```python
from build123d import *

# Parameters (mm, degrees)
SKETCH_1_R                   = 5
EXTRUDE_1_DEPTH              = 10.5
EXTRUDE_1_DEPTH_BACK         = 10.5
EXTRUDE_3_DEPTH              = 4.5
EXTRUDE_3_DEPTH_BACK         = 4.5
SKETCH_7_R                   = 6
EXTRUDE_4_DEPTH              = 3
SKETCH_8_R                   = 6
EXTRUDE_5_DEPTH              = 3
SKETCH_9_R                   = 9.5
CUT_EXTRUDE_1_DEPTH          = 7
SKETCH_10_R                  = 8.5
CUT_EXTRUDE_2_DEPTH          = 9
HOLE_WIZARD_M4_1_D           = 3.3
SKETCH_22_W                  = 47.656916312
SKETCH_22_H                  = 14.908676054
CUT_EXTRUDE_3_DEPTH          = 1111
SKETCH_23_R                  = 9.5
SKETCH_23_R_2                = 8.5
EXTRUDE_6_DEPTH              = 2
HOLE_WIZARD_M3_1_D           = 3.2
HOLE_WIZARD_M3_1_CBORE_D     = 6.5
HOLE_WIZARD_M3_1_CBORE_DEPTH = 3.4
PATTERN_CIRCULAR_1_COUNT     = 6
HOLE_WIZARD_M3_2_D           = 3.2
HOLE_WIZARD_M3_2_CBORE_D     = 6.5
HOLE_WIZARD_M3_2_CBORE_DEPTH = 3.4
PATTERN_LINEAR_1_COUNT       = 3
PATTERN_LINEAR_1_PITCH       = 70
PATTERN_LINEAR_1_COUNT_DIR2  = 2
PATTERN_LINEAR_1_PITCH_DIR2  = 10
SKETCH_31_R                  = 3.25
EXTRUDE_7_DEPTH              = 5.5


with BuildPart() as part:
    # Sketch 1 → Extrude 1 (new body, two sides)
    with BuildSketch(Plane(origin=(0, 0, 0), x_dir=(1, 0, 0), z_dir=(0, 1, 0))) as extrude_1_sk:
        Circle(SKETCH_1_R)
    extrude(amount=EXTRUDE_1_DEPTH)
    extrude(extrude_1_sk.sketch, amount=-EXTRUDE_1_DEPTH_BACK)

    # Sketch 6 → Extrude 3 (add, two sides)
    with BuildSketch(Plane(origin=(0, 0, 0), x_dir=(1, 0, 0), z_dir=(0, 1, 0))) as extrude_3_sk:
        with BuildLine():
            Line((-12.5, 0), (-12.5, -260))
            ThreePointArc((-12.5, -260), (0, -272.5), (12.5, -260))
            Line((12.5, -260), (12.5, 0))
            ThreePointArc((12.5, 0), (0, 12.5), (-12.5, 0))
        make_face()
    extrude(amount=EXTRUDE_3_DEPTH)
    extrude(extrude_3_sk.sketch, amount=-EXTRUDE_3_DEPTH_BACK)

    # Sketch 7 → Extrude 4 (add)
    with BuildSketch(Plane.XZ.offset(4.5)):
        Circle(SKETCH_7_R)
    extrude(amount=EXTRUDE_4_DEPTH)

    # Sketch 8 → Extrude 5 (add)
    with BuildSketch(Plane(origin=(0, 4.5, 0), x_dir=(1, 0, 0), z_dir=(0, 1, 0))):
        Circle(SKETCH_8_R)
    extrude(amount=EXTRUDE_5_DEPTH)

    # Sketch 9 → Cut-Extrude 1 (cut)
    with BuildSketch(Plane.XZ.offset(4.5)):
        with Locations((0, 250)):
            Circle(SKETCH_9_R)
    extrude(amount=-CUT_EXTRUDE_1_DEPTH, mode=Mode.SUBTRACT)

    # Sketch 10 → Cut-Extrude 2 (cut, through all)
    with BuildSketch(Plane.XZ.offset(-2.5)):
        with Locations((0, 250)):
            Circle(SKETCH_10_R)
    extrude(amount=-CUT_EXTRUDE_2_DEPTH, mode=Mode.SUBTRACT)

    # Hole Wizard M4 _ _ _ _1 (through all)
    with Locations(Plane(origin=(0, -10.5, 0), x_dir=(-1, 0, 0), z_dir=(0, -1, 0))):
        with Locations((0, 0)):
            Hole(HOLE_WIZARD_M4_1_D / 2)

    # Sketch 22 → Cut-Extrude 3 (cut, symmetric)
    with BuildSketch(Plane.XY):
        with Locations((0.455125877, 8.454338027)):
            Rectangle(SKETCH_22_W, SKETCH_22_H)
    extrude(amount=CUT_EXTRUDE_3_DEPTH, both=True, mode=Mode.SUBTRACT)

    # Sketch 23 → Extrude 6 (add)
    with BuildSketch(Plane.XZ.offset(4.5)):
        with Locations((0, 250)):
            Circle(SKETCH_23_R)
        with Locations((0, 250)):
            Circle(SKETCH_23_R_2, mode=Mode.SUBTRACT)
    extrude(amount=-EXTRUDE_6_DEPTH)

    # Hole Wizard M3 _ _ _ _ _ _1 (through all)
    with Locations(Plane(origin=(0, -4.5, 0), x_dir=(-1, 0, 0), z_dir=(0, -1, 0))):
        with Locations((6.75, -261.691342951)):
            hole_wizard_m3_1 = CounterBoreHole(HOLE_WIZARD_M3_1_D / 2, HOLE_WIZARD_M3_1_CBORE_D / 2, HOLE_WIZARD_M3_1_CBORE_DEPTH)

    # Pattern Circular 1: Hole Wizard M3 _ _ _ _ _ _1 ×6 about axis, 2 skipped
    pattern_circular_1_axis = Axis((0, -2.5, 250), (0, -1, 0))
    add([hole_wizard_m3_1.rotate(pattern_circular_1_axis, i * 360 / PATTERN_CIRCULAR_1_COUNT) for i in range(1, PATTERN_CIRCULAR_1_COUNT) if i not in (1, 4)], mode=Mode.SUBTRACT)

    # Hole Wizard M3 _ _ _ _ _ _2 (through all)
    with Locations(Plane(origin=(0, -4.5, 0), x_dir=(-1, 0, 0), z_dir=(0, -1, 0))):
        with Locations((5, -15)):
            hole_wizard_m3_2 = CounterBoreHole(HOLE_WIZARD_M3_2_D / 2, HOLE_WIZARD_M3_2_CBORE_D / 2, HOLE_WIZARD_M3_2_CBORE_DEPTH)

    # Pattern Linear 1: Hole Wizard M3 _ _ _ _ _ _2 3 × 2
    with Locations(*[(j * PATTERN_LINEAR_1_PITCH_DIR2, 0, i * PATTERN_LINEAR_1_PITCH) for i in range(PATTERN_LINEAR_1_COUNT) for j in range(PATTERN_LINEAR_1_COUNT_DIR2) if (i, j) != (0, 0)]):
        add(hole_wizard_m3_2, mode=Mode.SUBTRACT)

    # Sketch 31 → Extrude 7 (add)
    with BuildSketch(Plane.XZ.offset(4.5)):
        with Locations((5, 15)):
            Circle(SKETCH_31_R)
        with Locations((-5, 15)):
            Circle(SKETCH_31_R)
    extrude(amount=-EXTRUDE_7_DEPTH)


solid = part.part
```
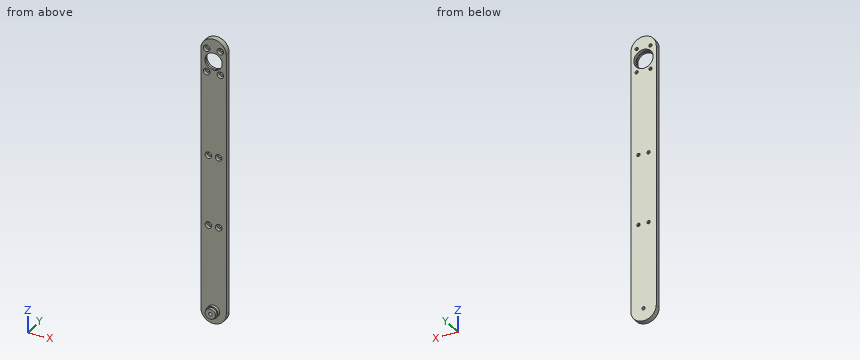
Work out the finished part from the listing and answer in its coordinate system (mm). Give positions to 0.01 mm unless a question says otherwise; leave off trailing zeros. Order: outer loops, then holes, each group sorted by start corner. A loop starts at its lowest first (then second) coordinate and runs counter-clockwise, first axis right, second up.
1. Each of these flat-tipped pins is pushed along its axis until it touches: P1, Ø3.5, axis at x = 5, z = 155, coming from the -Y side; P2, Ø4, axis at x = 0.5, z = 185, coming from the -Y side; P3, Ø2, axis at x = -10, y = -3.5, coming from the -Z side. Where does it stop, or does it pass through?
Result sheet:
P1: stops at y = -1.1
P2: stops at y = -4.5
P3: stops at z = -8.67
2. Section A-A, the plane z = 250 is taken. Determine the outline of the cut face in (x, y).
Result sheet:
outline: (-12.5, -4.5) - (-8.5, -4.5) - (-8.5, -2.5) - (-9.5, -2.5) - (-9.5, 1) - (-12.5, 1) - close; (8.5, -4.5) - (12.5, -4.5) - (12.5, 1) - (9.5, 1) - (9.5, -2.5) - (8.5, -2.5) - close
3. Straight lines are drawn through the part: L1, parallel to Z at x = 0, y = -0.75; L2, parallel to X at y = 0.3, z = 85; L3, parallel to Z at x = 8, y = -1.25. For each, find the intervals that lie inside material, in ascending order.
Result sheet:
L1: z = -12.5 to -1.65, 1.65 to 240.5, 259.5 to 272.5
L2: x = -12.5 to -6.6, -3.4 to 3.4, 6.6 to 12.5
L3: z = -9.6 to 83.75, 86.25 to 153.75, 156.25 to 235.31, 241.31 to 244.88, 255.12 to 258.69, 264.69 to 269.6
4. Section B-B, the plane z = 216.5 is taken. Determine the outline of the cut face in (x, y).
Result sheet:
outline: (-12.5, -4.5) - (12.5, -4.5) - (12.5, 1) - (-12.5, 1) - close
